Geometry check sheet. Reference: the model listing, model coordinates, mm. Face numbers are marked on the shaded views. A direction names the side the tool comes from. Coordinates: 2 decimals unless noted, no trailing zeros. Write each loop counter-clockwise with the first axis right and the second up, starting at its lowest first coordinate (ties: lowest second). Pieces come first, ordered by that corner, then holes.
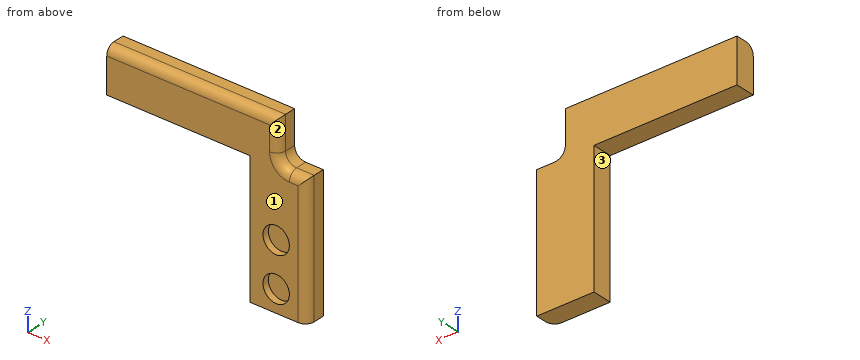
from build123d import *

# Parameters (mm, degrees)
EXTRUDE_1_DEPTH     = 9
FILLET_1_R          = 4
SKETCH_2_R          = 6
CUT_EXTRUDE_1_DEPTH = 3


with BuildPart() as part:
    # 草圖1 → 填料-伸長1 (new body)
    with BuildSketch(Plane(origin=(0, 0, 0), x_dir=(1, 0, 0), z_dir=(0, 1, 0))):
        with BuildLine():
            Line((0, 0), (65, 0))
            Line((65, 0), (65, 60))
            Line((65, 60), (91, 60))
            Line((91, 60), (91, 0))
            Line((91, 0), (83, 0))
            ThreePointArc((83, 0), (79.464466094, -1.464466094), (78, -5))
            Line((78, -5), (78, -20))
            Line((78, -20), (0, -20))
            Line((0, -20), (0, 0))
        make_face()
    extrude(amount=EXTRUDE_1_DEPTH)

    # 圓角1
    fillet_1_edges = [part.edges().sort_by_distance(p)[0] for p in [
        (87, 0, 0),
        (79.464466094, 0, 1.464466094),
        (78, 0, 12.5),
        (39, 0, 20),
        (91, 0, -30),
    ]]
    fillet(fillet_1_edges, radius=FILLET_1_R)

    # 草圖2 → 除料-伸長1 (cut)
    with BuildSketch(Plane.XZ):
        with Locations(Location((77, -50, 0), (0, 0, 270))):
            Circle(SKETCH_2_R)
        with Locations(Location((77, -30, 0), (0, 0, 270))):
            Circle(SKETCH_2_R)
    extrude(amount=-CUT_EXTRUDE_1_DEPTH, mode=Mode.SUBTRACT)


solid = part.part
1. Gauge pin test, flat ends, axial feed: pin 1 Ø9.5 at (x, z) = (77, -30) entering from -Y; pin 2 Ø1.5 at (y, z) = (5.5, 10) entering from +X; pin 3 Ø2.5 at (x, y) = (87.5, 6) entering from +Z. Record the tip position at first contact, or that the pin passes through.
Computed values:
pin 1: stops at y = 3
pin 2: stops at x = 78
pin 3: stops at z = 0
2. Sectioned sample at C-C, the plane z = 12. Record the boundary of the cut face in (x, y), and give its area (3 significant figures).
Computed values:
outline: (0, 0) - (74, 0) arc R4 ccw to (78, 4) - (78, 9) - (0, 9) - close
area: 699 mm2
3. Access from +Z, -Z, +X, -X, +Y, -Y to the whole of each face (thin tool, end or side, straight path). Record for the marked faces 1, 2 and 3.
Computed values:
face 1: +Z, -Z, +X, -X, -Y
face 2: +Z, +X, -Y
face 3: -Z, -X, +Y, -Y
4. Sectioned sample at B-B, the plane x = 62. Record the boundary of the cut face in (y, z).
Computed values:
outline: (0, 0) - (9, 0) - (9, 20) - (4, 20) arc R4 ccw to (0, 16) - close
5. Sectioned sample at A-A, the plane z = -30. Record the boundary of the cut face in (x, y).
Computed values:
outline: (65, 0) - (71, 0) - (71, 3) - (83, 3) - (83, 0) - (87, 0) arc R4 ccw to (91, 4) - (91, 9) - (65, 9) - close
6. Thickness scan on line 1 along X through (y, z) = (8.5, -49); line 2 along Z through (x, y) = (15, 8.5); line 3 along X through (y, z) = (0.8, -50). Record the ranges inside material, lowest first.
Computed values:
line 1: x = 65 to 91
line 2: z = 0 to 20
line 3: x = 65 to 71, 83 to 89.4
